The listing builds one solid part. Answer for the finished solid, in the listing's coordinates (mm). A direction names the side the tool comes from. Coordinates: 2 decimals unless noted, no trailing zeros. Loops run counter-clockwise (first coordinate to the right, second up) from the corner with the lowest first, then second, coordinate; pieces in that order, holes last. Notation, with made-up numbers: M -36,64.25 L 0,64.25 A22 cw 0,86.25 Z; hole C 28,-11 d7. An arc over 180 degrees is marked long. Answer as a JSON object with one key per item and string values. Group by question number.
1. For faces 1 (the face through (15.265, -380.822, 20.242)), 2 (the face through (1.81, -194.09, 1.91)), determine the directions among +Z, -Z, +X, -X, +Y, -Y from which every point of the face is accessible in a straight line to the end or side of a thin tool.
2. Straight lines are drawn through the part: L1, parallel to Z at x = 19.05, y = -373.5; L2, parallel to Z at x = 19.5, y = -315.5. For each, find the intervals that lie inside material, in ascending order.
3. Determine the mould class of faces 3 (the face through (15.085, -12.878, 19.224)), 4 (the face through (0, -194, 13)), 5 (the face through (23, 0, 15)), 6 (the face through (38.1, -194, 13)) for opening direction X: released by +X, released by -X, zero draft, split by the parting line, or undercut.
4. Given pin 1 (7 mm diameter, centred on x = 19.05, z = 19.05, fed in from -Y); pin 2 (6 mm diameter, centred on y = -266, z = 33.5, fed in from -X) (3 decimals); pin 3 (6.5 mm diameter, centred on x = 19.05, z = 19.05, fed in from -Y), each flat-ended and moving along its own axis, determine where each tip first touches the part or whether it passes through.
5. A cutting plane is placed at A-A on y = -40. Give the vertices of the cut face in (x, z), and give its area (3 significant figures).
6. A cutting plane is placed at B-B on x = 10.5. Give the vertices of the cut face in (y, z).
from build123d import *

# Parameters (mm, degrees)
F1_DEPTH       = 393.7
F4_D           = 7.9375
F4_DEPTH       = 25.4
F4_TIP         = 2.3846655818
F4_ON_F3_D     = 7.9375
F4_ON_F3_DEPTH = 25.4
F4_ON_F3_TIP   = 2.3846655818


with BuildPart() as f1:
    # F0 (on Front) → F1 (new body)
    with BuildSketch(Plane.XZ):
        with BuildLine():
            ThreePointArc((0, 6.35), (1.8598719395, 1.8598719395), (6.35, 0))
            Line((6.35, 0), (31.75, 0))
            ThreePointArc((31.75, 0), (36.2401280605, 1.8598719395), (38.1, 6.35))
            Line((38.1, 6.35), (38.1, 19.05))
            ThreePointArc((38.1, 19.05), (19.05, 38.1), (0, 19.05))
            Line((0, 19.05), (0, 6.35))
        make_face()
    extrude(amount=F1_DEPTH)

    # F4
    with Locations(Plane.XZ.offset(393.7)):
        with Locations((19.05, 19.05)):
            Hole(F4_D / 2, depth=F4_DEPTH)
            with Locations((0, 0, -(F4_DEPTH + F4_TIP / 2))):  # 118° drill point
                Cone(0, F4_D / 2, F4_TIP, mode=Mode.SUBTRACT)

    # F4 on F3
    with Locations(Plane(origin=(0, 0, 0), x_dir=(-1, 0, 0), z_dir=(0, 1, 0))):
        with Locations((-19.05, 19.05)):
            Hole(F4_ON_F3_D / 2, depth=F4_ON_F3_DEPTH)
            with Locations((0, 0, -(F4_ON_F3_DEPTH + F4_ON_F3_TIP / 2))):  # 118° drill point
                Cone(0, F4_ON_F3_D / 2, F4_ON_F3_TIP, mode=Mode.SUBTRACT)


solid = f1.part
From the geometry:
{
 "1": {"face 1": "-Y", "face 2": "-Z, -X, +Y, -Y"},
 "2": {"L1": "z = 0 to 15.08, 23.02 to 38.1", "L2": "z = 0 to 38.09"},
 "3": {"face 3": "undercut", "face 4": "released by -X", "face 5": "zero draft", "face 6": "released by +X"},
 "4": {"pin 1": "stops at y = -368.02", "pin 2": "stops at x = 3.825", "pin 3": "stops at y = -367.87"},
 "5": {"outline": "M 0,6.35 A6.35 ccw 6.35,0 L 31.75,0 A6.35 ccw 38.1,6.35 L 38.1,19.05 A19.05 ccw 0,19.05 Z", "area": "1,280 mm²"},
 "6": {"outline": "M -393.7,0 L 0,0 L 0,36.07 L -393.7,36.07 Z"}
}
